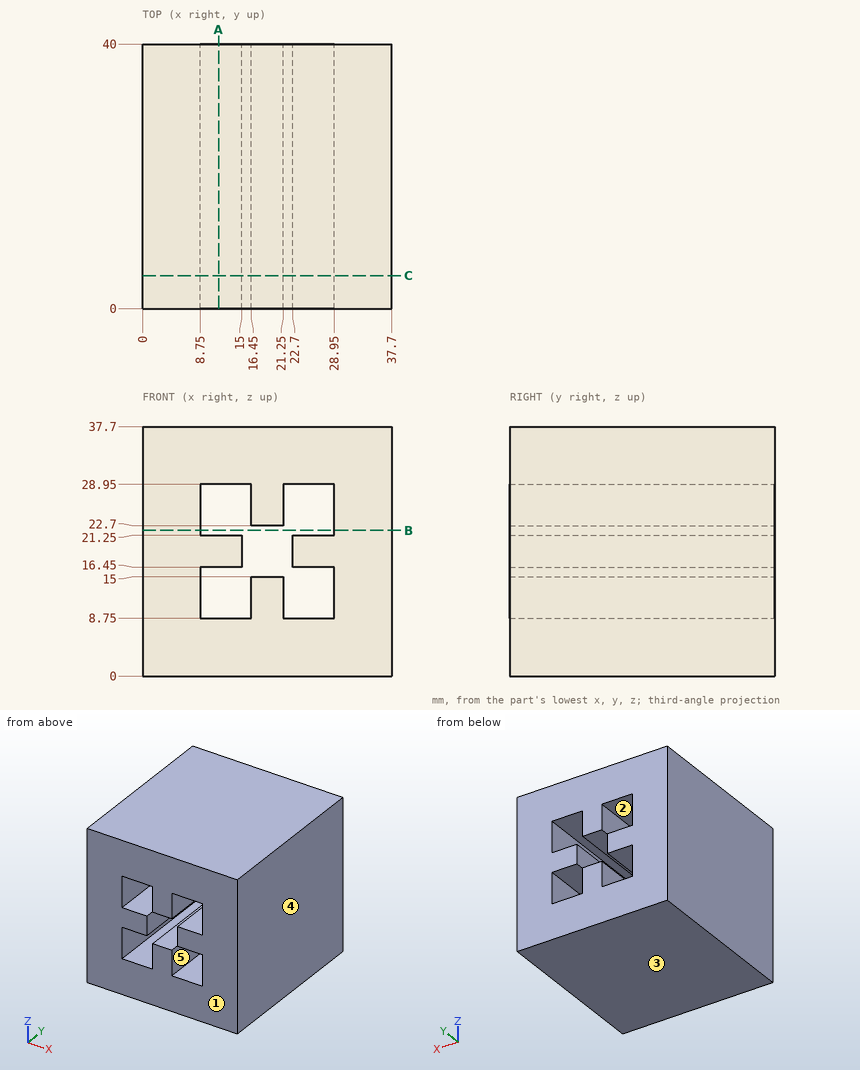
Check sheet for the drawn part. Datum: minimum x, y, z corner. Units: mm. A direction names the side the tool comes from. Give positions to 0.01 mm unless a question says otherwise; leave off trailing zeros. Write each loop counter-clockwise with the first axis right and the second up, starting at its lowest first coordinate (ties: lowest second). Pieces come first, ordered by that corner, then holes. Notation, with made-up numbers: (-12, 0) -> (7, 0) arc R17 ccw to (7, 17) -> close; hole circle Ø7 at (-0.75, 50). An arc over 180 degrees is marked (long way). Use one line per item in the form item = value. Start each with the question number.
1. Section check B-B (z = 22). Record the cut outline in (x, y).
2. Section check C-C (y = 5). Record the cut outline in (x, z), and give its area (3 significant figures).
3. Access from +Z, -Z, +X, -X, +Y, -Y to the whole of each face (thin tool, end or side, straight path). Record for the marked faces 1 and 2.
4. Mould release check, pull along Z, two halves, no side actions. Record for the marked faces 3, 4 and 5: pulls with the +Z half, pulls with the -Z half, needs draft (parallel to the pull), parting line crosses it, or undercut.
5. Thickness scan on line 1 along X through (y, z) = (30.5, 13.5); line 2 along X through (y, z) = (33.5, 20). Record the ranges inside material, lowest first. Write a range as from..to.
6. Section check A-A (x = 11.5). Record the cut outline in (y, z), and give its area (3 significant figures).
Conclusion:
q1.outline = (0, 0) -> (8.75, 0) -> (8.75, 40) -> (0, 40) -> close; (28.95, 0) -> (37.7, 0) -> (37.7, 40) -> (28.95, 40) -> close
q2.outline = (0, 0) -> (37.7, 0) -> (37.7, 37.7) -> (0, 37.7) -> close; hole (8.75, 8.75) -> (16.45, 8.75) -> (16.45, 15) -> (21.25, 15) -> (21.25, 8.75) -> (28.95, 8.75) -> (28.95, 16.45) -> (22.7, 16.45) -> (22.7, 21.25) -> (28.95, 21.25) -> (28.95, 28.95) -> (21.25, 28.95) -> (21.25, 22.7) -> (16.45, 22.7) -> (16.45, 28.95) -> (8.75, 28.95) -> (8.75, 21.25) -> (15, 21.25) -> (15, 16.45) -> (8.75, 16.45) -> close
q2.area = 1,130 mm²
q3.face_1 = +Z, -Z, +X, -X, -Y
q3.face_2 = +Y, -Y
q4.face_3 = pulls with the -Z half
q4.face_4 = needs draft
q4.face_5 = undercut
q5.line_1 = 0..8.75, 16.45..21.25, 28.95..37.7
q5.line_2 = 0..15, 22.7..37.7
q6.outline = (0, 0) -> (40, 0) -> (40, 8.75) -> (0, 8.75) -> close; (0, 16.45) -> (40, 16.45) -> (40, 21.25) -> (0, 21.25) -> close; (0, 28.95) -> (40, 28.95) -> (40, 37.7) -> (0, 37.7) -> close
q6.area = 892 mm²
